```python
from build123d import *

# Parameters (mm, degrees)
F0_R      = 9
F1_DEPTH  = 14
F2_R      = 6
F3_DEPTH  = 22
F4_R      = 5.55
F5_DEPTH  = 1.15
F6_R      = 6
F7_DEPTH  = 3.5
F8_R      = 5
F9_DEPTH  = 9.5
F10_SIZE  = 0.5
F11_SIZE  = 1
F13_D     = 6
F13_DEPTH = 22
F13_TIP   = 1.8025818571
F15_D     = 5.5
F15_DEPTH = 22
F15_TIP   = 1.6523667023


with BuildPart() as f1:
    # F0 (on Top) → F1 (new body)
    with BuildSketch(Plane.XY):
        Circle(F0_R)
    extrude(amount=F1_DEPTH)

    # F2 (on face) → F3 (join)
    with BuildSketch(Plane(origin=(0, 0, 0), x_dir=(1, 0, 0), z_dir=(0, 0, -1))):
        Circle(F2_R)
    extrude(amount=F3_DEPTH)

    # F4 (on face) → F5 (join)
    with BuildSketch(Plane(origin=(0, 0, -22), x_dir=(1, 0, 0), z_dir=(0, 0, -1))):
        Circle(F4_R)
    extrude(amount=F5_DEPTH)

    # F6 (on face) → F7 (join)
    with BuildSketch(Plane(origin=(0, 0, -23.15), x_dir=(1, 0, 0), z_dir=(0, 0, -1))):
        Circle(F6_R)
    extrude(amount=F7_DEPTH)

    # F8 (on face) → F9 (join)
    with BuildSketch(Plane(origin=(0, 0, -26.65), x_dir=(1, 0, 0), z_dir=(0, 0, -1))):
        Circle(F8_R)
    extrude(amount=F9_DEPTH)

    # F10
    f10_edges = [f1.edges().sort_by_distance(p)[0] for p in [
        (-5, 0, -36.15),
    ]]
    chamfer(f10_edges, length=F10_SIZE)

    # F11
    f11_edges = [f1.edges().sort_by_distance(p)[0] for p in [
        (-9, 0, 14),
    ]]
    chamfer(f11_edges, length=F11_SIZE)

    # F13
    with Locations(Plane.XY.offset(14)):
        with Locations((0, 0)):
            Hole(F13_D / 2, depth=F13_DEPTH)
            with Locations((0, 0, -(F13_DEPTH + F13_TIP / 2))):  # 118° drill point
                Cone(0, F13_D / 2, F13_TIP, mode=Mode.SUBTRACT)

    # F15 (one way)
    with BuildSketch(Plane(origin=(0, 0, 0), x_dir=(1, 0, 0), z_dir=(0, 1, 0))):
        with Locations((0, -6)):
            Circle(F15_D / 2)
    extrude(amount=-F15_DEPTH, mode=Mode.SUBTRACT)
    with Locations(Plane(origin=(0, 0, 0), x_dir=(1, 0, 0), z_dir=(0, 1, 0))):
        with Locations((0, -6)):
            with Locations((0, 0, -(F15_DEPTH + F15_TIP / 2))):  # 118° drill point
                Cone(0, F15_D / 2, F15_TIP, mode=Mode.SUBTRACT)


solid = f1.part
```
Verification items for the finished model (mm, model axes). A direction names the side the tool comes from. Coordinates: 2 decimals unless noted, no trailing zeros. Order: outer loops, then holes, each group sorted by start corner. A loop starts at its lowest first (then second) coordinate and runs counter-clockwise, first axis right, second up. Notation, with made-up numbers: (28.5, 20) -> (78.5, 20) arc R17 ccw to (78.5, 42) -> close; hole circle Ø1 at (86.5, -5). An arc over 180 degrees is marked (long way). Put each result on its own line as item: value. Start each with the question number.
1) Go/stop test with flat-tipped pins: pin 1 (2 mm diameter, centred on x = -4.5, z = -10, fed in from -Y); pin 2 (3 mm diameter, centred on y = 4.5, z = -18, fed in from -X); pin 3 (2 mm diameter, centred on x = -2, z = -24.5, fed in from -Y). Record where each tip stops, or that it passes through.
2) Cross-section at C-C (z = 6). Enter the section's corners in (x, y), plus the area to 3 significant figures.
3) Material ranges on L1, parallel to X at y = 0, z = -3.5; L2, parallel to Z at x = 0, y = -5.5, recorded low to high.
4) Cross-section at A-A (z = -0.5). Enter the section's corners in (x, y).
5) Release check for a two-part mould opening along Y. For faces 6 (the cylindrical face through (2.98, -4.68, -22.57)), 7 (the cylindrical face through (0, 3, 3)), 8 (the flat face through (-3, 5, -22)) record: pulls with the +Y half, pulls with the -Y half, needs draft (parallel to the pull), parting line crosses it, or undercut.
6) Cross-section at B-B (z = -21). Enter the section's corners in (x, y), plus the area to 3 significant figures.
7) Tool access check on faces 1 (the flat face through (3.4, 0.1, 14)), 2 (the flat face through (-3, 5, -23.15)), 3 (the cylindrical face through (-1.172, 8.923, 6.409)), 4 (the cylindrical face through (-2.027, -5.913, 4.141)), 5 (the cylindrical face through (-6, 0, -25)). Record the directions out of +Z, -Z, +X, -X, +Y, -Y that give a thin tool (end or side, any length) a straight path to the whole face; none if there is none.
Geometry check:
1. pin 1: stops at y = -4.87
1. pin 2: stops at x = -5.2
1. pin 3: stops at y = -5.92
2. outline: (-2.75, -8.57) -> (-2.75, -1.2) arc R3 cw (long way) to (2.75, -1.2) -> (2.75, -8.57) arc R9 ccw (long way) to start
2. area: 191 mm^2
3. L1: x = -6 to -3, 3 to 6
3. L2: z = -26.65 to 3.25, 8.75 to 14
4. outline: circle Ø12 at (0, 0); hole circle Ø6 at (0, 0)
5. face 6: parting line crosses it
5. face 7: undercut
5. face 8: needs draft
6. outline: circle Ø12 at (0, 0)
6. area: 113 mm^2
7. face 1: +Z, +X, -X, +Y, -Y
7. face 2: none
7. face 3: +Z, -Z
7. face 4: -Y
7. face 5: -Z
